from build123d import *

# Parameters (mm, degrees)
F1_DEPTH  = 16
F2_W      = 70
F2_H      = 3
F3_DEPTH  = 2
F4_W      = 50
F4_H      = 14
F5_DEPTH  = 2
F6_R      = 1
F9_DEPTH  = 2
F11_DEPTH = 38.001
F13_D     = 4
F14_R     = 3
F14_R_2   = 2
F15_DEPTH = 5
F16_R     = 3


# Not quite as in the source:
# - a pattern or mirror of a feature is missing from the dataset's text; its kind, count and spacing are read off the source's solid


with BuildPart() as f1:
    # F0 (on Front) → F1 (new body)
    with BuildSketch(Plane.XZ):
        with BuildLine():
            Line((94, 11), (0, 11))
            ThreePointArc((0, 11), (-11, 0), (0, -11))
            Line((0, -11), (19, -11))
            ThreePointArc((19, -11), (21.7681124643, -11.8361612201), (23.6103896104, -14.064978646))
            ThreePointArc((23.6103896104, -14.064978646), (47.381548553, -44.2322797447), (83.2800086179, -57.8863860143))
            ThreePointArc((83.2800086179, -57.8863860143), (88.6838234672, -59.2161173312), (93.142692854, -62.5459647892))
            Line((93.142692854, -62.5459647892), (94.4399113384, -61))
            ThreePointArc((94.4399113384, -61), (90.012513527, -57.6415445278), (84.7034264019, -56))
            ThreePointArc((84.7034264019, -56), (49.0672193413, -42.9854179344), (25.4545454545, -13.2909701044))
            ThreePointArc((25.4545454545, -13.2909701044), (22.87535745, -10.1706257081), (19, -9))
            Line((19, -9), (0, -9))
            ThreePointArc((0, -9), (-9, 0), (0, 9))
            Line((0, 9), (94, 9))
            Line((94, 9), (94, 11))
        make_face()
    extrude(amount=F1_DEPTH)

    # F2 (on face) → F3 (join)
    with BuildSketch(Plane.XY.offset(11)):
        with Locations((59, -17.5)):
            Rectangle(F2_W, F2_H)
    extrude(amount=-F3_DEPTH)

    # F4 (on face) → F5 (join)
    with BuildSketch(Plane.XZ.offset(19)):
        with Locations((69, 4)):
            Rectangle(F4_W, F4_H)
    extrude(amount=-F5_DEPTH)

    # F6
    f6_edges = [f1.edges().sort_by_distance(p)[0] for p in [
        (44, -18, 9),
    ]]
    fillet(f6_edges, radius=F6_R)

    # F7: F1 across plane


with BuildPart() as f1_1:
    add(f1.part)
    add(f1.part.mirror(Plane.XZ))

    # F8 (on face) → F9 (cut)
    with BuildSketch(Plane.XY.offset(11)):
        with BuildLine():
            Line((94, 12), (34, 12))
            ThreePointArc((34, 12), (22, 0), (34, -12))
            Line((34, -12), (94, -12))
            Line((94, -12), (94, 12))
        make_face()
    extrude(amount=-F9_DEPTH, mode=Mode.SUBTRACT)

    # F10 (on face) → F11 (cut, through all)
    with BuildSketch(Plane.XZ.offset(19)):
        with BuildLine():
            ThreePointArc((50, 5), (47, 2), (50, -1))
            Line((50, -1), (70, -1))
            ThreePointArc((70, -1), (73, 2), (70, 5))
            Line((70, 5), (50, 5))
        make_face()
    extrude(amount=-F11_DEPTH, mode=Mode.SUBTRACT)

    # F13 (through all)
    with Locations(Plane.XZ.offset(19)):
        with Locations((80, 3)):
            Hole(F13_D / 2)

    # F14 (on face) → F15 (join)
    with BuildSketch(Plane(origin=(0, -17, 0), x_dir=(-1, 0, 0), z_dir=(0, 1, 0))):
        with Locations((-80, 3)):
            Circle(F14_R)
        with Locations((-80, 3)):
            Circle(F14_R_2, mode=Mode.SUBTRACT)
    f15 = extrude(amount=F15_DEPTH)

    # F15_copies: F15 across plane
    add(f15.mirror(Plane.ZX))

    # F16
    f16_edges = [f1_1.edges().sort_by_distance(p)[0] for p in [
        (94, -18, -3),
        (44, -18, -3),
        (94, 18, -3),
        (44, 18, -3),
    ]]
    fillet(f16_edges, radius=F16_R)


solid = f1_1.part
Geometry check sheet. Reference: the model listing, model coordinates, mm. A direction names the side the tool comes from. Give positions to 0.01 mm unless a question says otherwise; leave off trailing zeros. Loops run counter-clockwise (first coordinate to the right, second up) from the corner with the lowest first, then second, coordinate; pieces in that order, holes last. Notation, with made-up numbers: M 74,76.25 L 81,76.25 A19 ccw 81,87.25 Z; hole C 37.25,30 d5. An arc over 180 degrees is marked long. Answer as a JSON object with one key per item and string values. Group by question number.
Item 1: Mould release check, pull along Y, two halves, no side actions. Record for faces 6 (the cylindrical face through (49.505, -0.224, -43.298)), 7 (the flat face through (30, -16, -23)), 8 (the flat face through (35.9, 12.4, 9)): pulls with the +Y half, pulls with the -Y half, needs draft (parallel to the pull), parting line crosses it, or undercut.
Item 2: Gauge pin test, flat ends, axial feed: pin 1 (2 mm diameter, centred on x = 65.5, y = 17.5, fed in from -Z); pin 2 (2 mm diameter, centred on y = 18, z = 3, fed in from -X); pin 3 (1.6 mm diameter, centred on y = 18, z = 10.5, fed in from -X); pin 4 (6 mm diameter, centred on x = 79, z = -8, fed in from +Y). Record the tip position at first contact, or that the pin passes through.
Item 3: Sectioned sample at B-B on y = 0. Record the boundary of the cut face in (x, z), plus the area to 3 significant figures.
Item 4: Access from +Z, -Z, +X, -X, +Y, -Y to the whole of each face (thin tool, end or side, straight path). Record for faces 1 (the cylindrical face through (78.092, 15.549, 3.601)), 2 (the flat face through (79, -12, 1)), 3 (the cylindrical face through (90.082, -0.224, -57.677)), 4 (the flat face through (94, -18, 7)), 5 (the cylindrical face through (83, 15, 3)).
Item 5: Sectioned sample at A-A on x = 16.5. Record the boundary of the cut face in (y, z), plus the area to 3 significant figures.
Item 6: Sectioned sample at C-C on x = 88. Record the boundary of the cut face in (y, z).
Item 7: Material ranges on L1, parallel to Z at x = 80, y = 16.25; L2, parallel to Z at x = 10, y = 0.5; L3, parallel to Y at x = 82.5, z = -1, recorded low to high.
Item 8: Sectioned sample at D-D on z = 3. Give the number of separate pieces and of enclosed holes in the cut face, plus the area to 4 significant figures.
Findings below:
{
 "1": {"face 6": "needs draft", "face 7": "pulls with the -Y half", "face 8": "undercut"},
 "2": {"pin 1": "z = -3", "pin 2": "x = 44", "pin 3": "x = 24", "pin 4": "through"},
 "3": {"outline": "M 0,-11 L 19,-11 A5 cw 23.61,-14.06 A72 ccw 83.28,-57.89 A14 cw 93.14,-62.55 L 94.44,-61 A16 ccw 84.7,-56 A70 cw 25.45,-13.29 A7 ccw 19,-9 L 0,-9 A9 cw 0,9 L 22,9 L 22,11 L 0,11 A11 ccw Z", "area": "336 mm2"},
 "4": {"face 1": "+Y, -Y", "face 2": "+Z, +X", "face 3": "+X, +Y, -Y", "face 4": "+Z, +X, +Y, -Y", "face 5": "none"},
 "5": {"outline": "M -16,-11 L 16,-11 L 16,-9 L -16,-9 Z; M -16,9 L 16,9 L 16,11 L -16,11 Z", "area": "128 mm2"},
 "6": {"outline": "M -19,-3 L -17,-3 L -17,9 L -12,9 L -12,11 L -19,11 Z; M -16,-58.92 L 16,-58.92 L 16,-56.78 L -16,-56.78 Z; M 12,9 L 17,9 L 17,-3 L 19,-3 L 19,11 L 12,11 Z"},
 "7": {"L1": "0 to 1, 5 to 6, 9 to 11", "L2": "-11 to -9, 9 to 11", "L3": "-19 to -17, 17 to 19"},
 "8": {"separate pieces": "7", "enclosed holes": "0", "area": "168.5 mm2"}
}
